The listing builds one solid part. Answer for the finished solid, in the listing's coordinates (mm). A direction names the side the tool comes from. Give positions to 0.01 mm unless a question says otherwise; leave off trailing zeros. Write each loop counter-clockwise with the first axis right and the second up, starting at its lowest first coordinate (ties: lowest second). Pieces come first, ordered by that corner, then holes. Notation, with made-up numbers: M 15,35 L 49,35 A34 cw 49,67 Z; hole C -33,10.5 d10. An arc over 180 degrees is marked long. Return JSON: item names as keys, results as strings.
from build123d import *

# Parameters (mm, degrees)
F0_R     = 0.75
F0_R_2   = 0.53
F1_DEPTH = 1


# Not quite as in the source:
# - a feature names something its author has since deleted; it is built from what else it names


with BuildPart() as f1:
    # F0 (on Right) → F1 (new body)
    with BuildSketch(Plane.YZ):
        Polygon((1.75, 0), (0, 0), (0, -11.5), (11.5, -11.5), (11.5, 0), (10.384144865, 0), (10.384144865, 10), (8.384144865, 10), (8.384144865, 0), (7.7499999977, 0), (5.750004947, 0), (3.75, 0), align=None)
        with Locations((1.7500000088, -9.75)):
            Circle(F0_R, mode=Mode.SUBTRACT)
        with Locations((1.75, -7.75)):
            Circle(F0_R, mode=Mode.SUBTRACT)
        with Locations((3.7499851588, -10.5567658602)):
            Circle(F0_R_2, mode=Mode.SUBTRACT)
        Polygon((5.3081902647, -9.0000098941), (5.7499752647, -9.0000098941), (6.1917602647, -9.0000098941), (6.4146452647, -9.0000098941), (6.4146452647, -10.3293498941), (6.1917602647, -10.3293498941), (5.0853052647, -10.3293498941), (5.0853052647, -9.0000098941), align=None, mode=Mode.SUBTRACT)
        Polygon((3.1706485936, -8.0853299912), (4.3492385936, -8.0853299912), (4.3492385936, -8.7499999912), (4.3492385936, -9.4146699912), (3.1706485936, -9.4146699912), (3.0198985936, -9.4146699912), (3.0198985936, -8.7499999912), (3.0198985936, -8.0853299912), align=None, mode=Mode.SUBTRACT)
        with Locations((3.7499923957, -6.75)):
            Circle(F0_R, mode=Mode.SUBTRACT)
        Polygon((6.4146452647, -8.5000098941), (5.7499752647, -8.5000098941), (5.0853052647, -8.5000098941), (5.0853052647, -7.1706698941), (6.1917602647, -7.1706698941), (6.4146452647, -7.1706698941), align=None, mode=Mode.SUBTRACT)
        with Locations((1.75, -5.75)):
            Circle(F0_R, mode=Mode.SUBTRACT)
        with Locations((1.75, -3.75)):
            Circle(F0_R, mode=Mode.SUBTRACT)
        with BuildLine():
            ThreePointArc((2.5, -1.75), (1.2196699141, -2.2803300859), (1.75, -1))
            ThreePointArc((1.75, -1), (2.2803300859, -1.2196699141), (2.5, -1.75))
        make_face(mode=Mode.SUBTRACT)
        with Locations((3.7499961979, -4.75)):
            Circle(F0_R, mode=Mode.SUBTRACT)
        with Locations((5.7499851588, -5.7500098941)):
            Circle(F0_R, mode=Mode.SUBTRACT)
        with Locations((5.7499950529, -3.7500098941)):
            Circle(F0_R, mode=Mode.SUBTRACT)
        with Locations((3.75, -2.75)):
            Circle(F0_R, mode=Mode.SUBTRACT)
        with BuildLine():
            ThreePointArc((4.28, -0.94325), (3.375233406, -1.318016594), (3.75, -0.41325))
            ThreePointArc((3.75, -0.41325), (4.124766594, -0.568483406), (4.28, -0.94325))
        make_face(mode=Mode.SUBTRACT)
        with Locations((7.749955461, -10.5567658602)):
            Circle(F0_R_2, mode=Mode.SUBTRACT)
        Polygon((7.1507119358, -8.7499999912), (7.1507119358, -8.0853299912), (8.3293019358, -8.0853299912), (8.4800519358, -8.0853299912), (8.4800519358, -8.7499999912), (8.4800519358, -9.4146699912), (8.3293019358, -9.4146699912), (7.1507119358, -9.4146699912), align=None, mode=Mode.SUBTRACT)
        with Locations((7.7499680167, -6.7500197925)):
            Circle(F0_R, mode=Mode.SUBTRACT)
        with Locations((9.7499307145, -9.750039585)):
            Circle(F0_R, mode=Mode.SUBTRACT)
        with Locations((9.749950516, -7.7500395851)):
            Circle(F0_R, mode=Mode.SUBTRACT)
        with Locations((7.7499840072, -4.7500197926)):
            Circle(F0_R, mode=Mode.SUBTRACT)
        with BuildLine():
            ThreePointArc((6.500004947, -1.7500098941), (5.2196748611, -2.28033998), (5.750004947, -1.0000098941))
            ThreePointArc((5.750004947, -1.0000098941), (6.2803350329, -1.2196798082), (6.500004947, -1.7500098941))
        make_face(mode=Mode.SUBTRACT)
        with Locations((7.7499999977, -2.7500197927)):
            Circle(F0_R, mode=Mode.SUBTRACT)
        with BuildLine():
            ThreePointArc((8.2799999977, -0.9432697927), (7.3752334037, -1.3180363867), (7.7499999977, -0.4132697927))
            ThreePointArc((7.7499999977, -0.4132697927), (8.1247665918, -0.5685031986), (8.2799999977, -0.9432697927))
        make_face(mode=Mode.SUBTRACT)
        with Locations((9.7499703087, -5.7500395852)):
            Circle(F0_R, mode=Mode.SUBTRACT)
        with Locations((9.7499901013, -3.7500395853)):
            Circle(F0_R, mode=Mode.SUBTRACT)
        with BuildLine():
            ThreePointArc((9.750009894, -1.0000395854), (10.2803399799, -1.2197094995), (10.500009894, -1.7500395854))
            ThreePointArc((10.500009894, -1.7500395854), (9.2196798081, -2.2803696712), (9.750009894, -1.0000395854))
        make_face(mode=Mode.SUBTRACT)
    extrude(amount=F1_DEPTH)


solid = f1.part
Item 1: A cutting plane is placed at B-B, the plane y = 2.75. Write down the section's boundary in (x, z), plus the area to 3 significant figures.
Geometry results:
{"outline": "M 0,-11.5 L 1,-11.5 L 1,0 L 0,0 Z", "area": "11.5 mm2"}
Item 2: A cutting plane is placed at A-A, the plane z = 0.75. Write down the section's boundary in (x, y).
Geometry results:
{"outline": "M 0,8.38 L 1,8.38 L 1,10.38 L 0,10.38 Z"}
Item 3: Which of the six approach directions +Z, -Z, +X, -X, +Y, -Y give full straight-line access (tool end or side, diameter ignored) to faces 4 (the flat face through (0.5, 11.5, -5.8)), 5 (the flat face through (0.5, 4.3, 0)), 6 (the flat face through (0.5, 5.7, -7.171))?
Geometry results:
{"face 4": "+Z, -Z, +X, -X, +Y", "face 5": "+Z, +X, -X, -Y", "face 6": "+X, -X"}
Item 4: Given pin 1 Ø2 at (y, z) = (5, -0.5) entering from -X; pin 2 Ø0.5 at (x, y) = (0.5, 3.5) entering from +Z, each flat-ended and moving along its own axis, determine where each tip first touches the part or whether it passes through.
Geometry results:
{"pin 1": "stops at x = 0", "pin 2": "stops at z = 0"}
Item 5: Determine the mould class of faces 1 (the flat face through (0, 6.9, -5.4)), 2 (the flat face through (0.5, 10.9, 0)), 3 (the cylindrical face through (0.493, 9.155, -8.206)) for opening direction Z: +Z half, -Z half, draft (parallel to the pull), parting line (faces both ways), or undercut.
Geometry results:
{"face 1": "draft", "face 2": "+Z half", "face 3": "undercut"}
Item 6: Find the intervals of material crossed by line 1 (Z direction, x = 0.15, y = 1.5); line 2 (Z direction, x = 0.55, y = 9.5); line 3 (Y direction, x = 0.4, z = -8), in increasing order.
Geometry results:
{"line 1": "z = -11.5 to -10.46, -9.04 to -8.46, -7.04 to -6.46, -5.04 to -4.46, -3.04 to -2.46, -1.04 to 0", "line 2": "z = -11.5 to -10.46, -9.04 to -8.46, -7.04 to -6.46, -5.04 to -4.46, -3.04 to -2.46, -1.04 to 10", "line 3": "y = 0 to 1.04, 2.46 to 5.09, 6.41 to 9.04, 10.46 to 11.5"}
Item 7: A cutting plane is placed at C-C, the plane x = 0.25. Count the separate pieces of the cut face and the enclosed holes in it, plus the area to 3 significant figures.
Geometry results:
{"separate pieces": "1", "enclosed holes": "27", "area": "108 mm2"}
